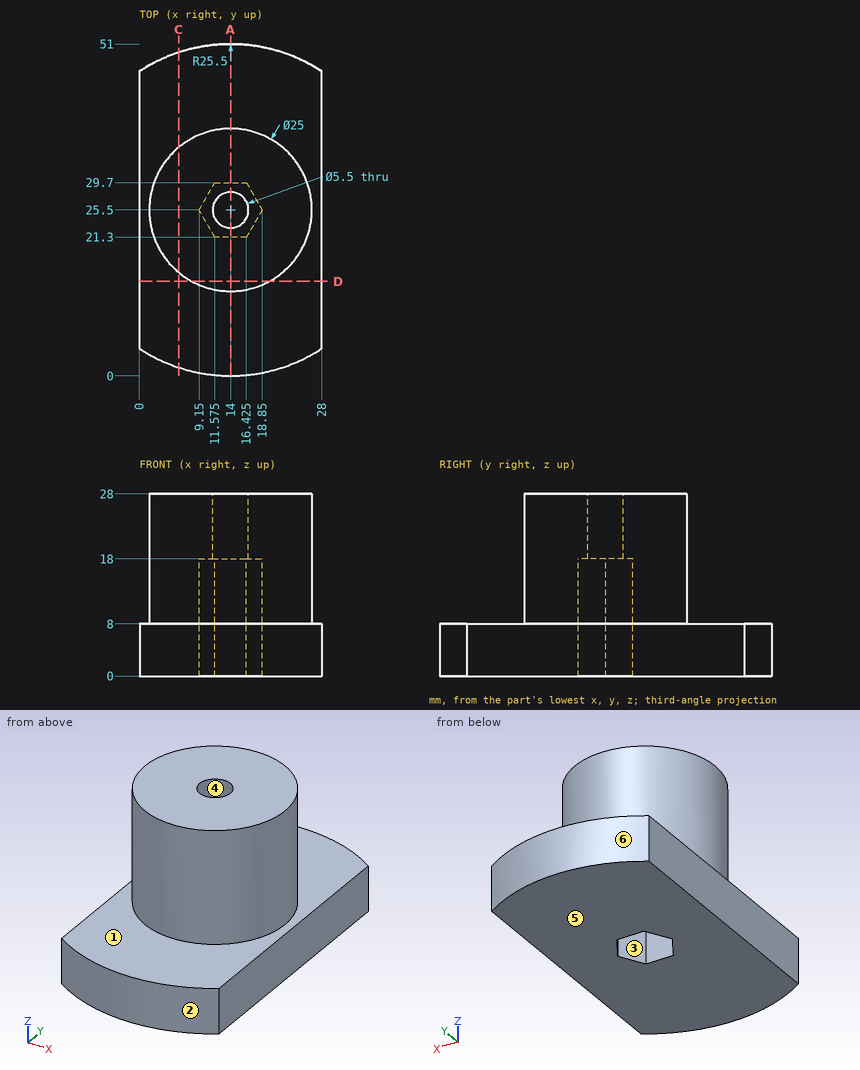
Geometry check sheet. Reference: drawing and pictorial views, mm from the part's lowest x, y, z. A direction names the side the tool comes from. Coordinates: 2 decimals unless noted, no trailing zeros. Write each loop counter-clockwise with the first axis right and the second up, starting at its lowest first coordinate (ties: lowest second). Pieces come first, ordered by that corner, then holes. Notation, with made-up numbers: (-9, -30) -> (45, -30) arc R37 cw to (45, 9) -> close; hole circle Ø2 at (-20.75, 79). An arc over 180 degrees is marked (long way). One line per question, with ' | ' between items.
1. Draft check along X on the marked faces 4, 5 and 6. Enter one of: +X half, -X half, draft (parallel to the pull), parting line (faces both ways), or undercut.
Answers:
face 4: undercut | face 5: draft | face 6: parting line
2. Thickness scan on probe 1 along X at (y, z) = (25.5, 23.25); probe 2 along Z at (x, y) = (23.5, 16.5); probe 3 along Y at (x, z) = (16, 22.5). Record the ranges inside material, lowest first. Write a range as from..to.
Answers:
probe 1: x = 1.5..11.25, 16.75..26.5 | probe 2: z = 0..8 | probe 3: y = 13.16..23.61, 27.39..37.84
3. Depth check by flat-ended pin: pin 1 Ø5.5 at (x, z) = (14, 13.5) entering from +Y; pin 2 Ø2.5 at (x, z) = (15, 11) entering from -Y; pin 3 Ø5 at (x, y) = (14, 42) entering from +Z. Enter the tip coordinate at first touch or a pass-through.
Answers:
pin 1: stops at y = 38 | pin 2: stops at y = 13 | pin 3: stops at z = 8
4. Cross-section at A-A on x = 14. Record the cut outline in (y, z), and give its area (3 significant figures).
Answers:
outline: (0, 0) -> (21.3, 0) -> (21.3, 18) -> (22.75, 18) -> (22.75, 28) -> (13, 28) -> (13, 8) -> (0, 8) -> close; (28.25, 18) -> (29.7, 18) -> (29.7, 0) -> (51, 0) -> (51, 8) -> (38, 8) -> (38, 28) -> (28.25, 28) -> close | area: 702 mm²
5. Cross-section at D-D on y = 14.5. Record the cut outline in (x, z).
Answers:
outline: (0, 0) -> (28, 0) -> (28, 8) -> (19.94, 8) -> (19.94, 28) -> (8.06, 28) -> (8.06, 8) -> (0, 8) -> close
6. Cross-section at C-C on x = 6. Record the cut outline in (y, z) (1 decimal).
Answers:
outline: (1.3, 0) -> (49.7, 0) -> (49.7, 8) -> (35.1, 8) -> (35.1, 28) -> (15.9, 28) -> (15.9, 8) -> (1.3, 8) -> close
7. Set-up check for the marked faces 1, 2 and 3: record each of +Z, -Z, +X, -X, +Y, -Y from which the full face is reachable in a straight line by a thin tool's end or side.
Answers:
face 1: +Z | face 2: +Z, -Z, -Y | face 3: -Z
